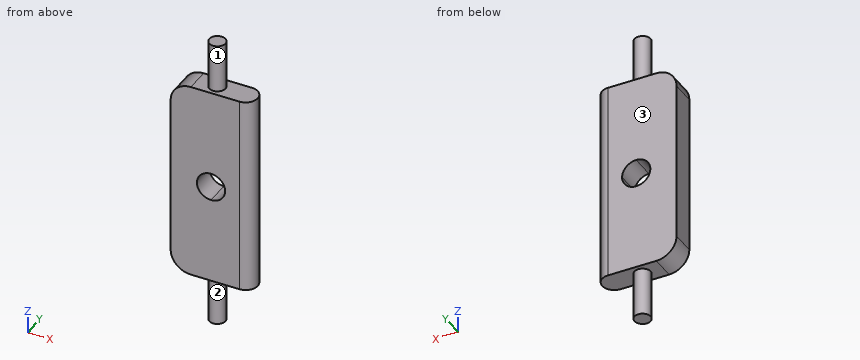
from build123d import *

# Parameters (mm, degrees)
SKETCH1_W           = 20
SKETCH1_H           = 50
BOSS_EXTRUDE1_DEPTH = 6
CUT_EXTRUDE1_DEPTH  = 55.184868737
BOSS_EXTRUDE2_DEPTH = 4
BOSS_EXTRUDE3_START = 4
BOSS_EXTRUDE3_DEPTH = 4
BOSS_EXTRUDE4_START = 1
SKETCH5_R           = 2
BOSS_EXTRUDE4_DEPTH = 1
SKETCH6_R           = 2
BOSS_EXTRUDE5_DEPTH = 1
FILLET1_R           = 5
FILLET2_R           = 5
FILLET3_RADIUS      = 3
FILLET3_LENGTH      = 50
BOSS_EXTRUDE6_START = 7
SKETCH7_R           = 2
BOSS_EXTRUDE6_DEPTH = 7
SKETCH8_R           = 2
BOSS_EXTRUDE7_DEPTH = 7


with BuildPart() as part:
    # Sketch1 → Boss-Extrude1 (new body)
    with BuildSketch(Plane(origin=(0, 0, 0), x_dir=(1, 0, 0), z_dir=(0, 1, 0))):
        with Locations((10, 25)):
            Rectangle(SKETCH1_W, SKETCH1_H)
    extrude(amount=BOSS_EXTRUDE1_DEPTH)

    # Sketch2 → Cut-Extrude1 (cut, through all)
    with BuildSketch(Plane(origin=(0, 6, 0), x_dir=(1, 0, 0), z_dir=(0, 1, 0))):
        with BuildLine():
            ThreePointArc((13.5, 25), (12.474873734, 27.474873734), (10, 28.5))
            Line((10, 28.5), (10, 21.5))
            ThreePointArc((10, 21.5), (12.474873734, 22.525126266), (13.5, 25))
        make_face()
        with BuildLine():
            Line((10, 21.5), (10, 28.5))
            ThreePointArc((10, 28.5), (6.5, 25), (10, 21.5))
        make_face()
    extrude(amount=-CUT_EXTRUDE1_DEPTH, mode=Mode.SUBTRACT)

    # Sketch3 → Boss-Extrude2 (add)
    with BuildSketch(Plane.XY):
        with BuildLine():
            ThreePointArc((12, 3), (11.414213562, 4.414213562), (10, 5))
            Line((10, 5), (10, 1))
            ThreePointArc((10, 1), (11.414213562, 1.585786438), (12, 3))
        make_face()
        with BuildLine():
            Line((10, 1), (10, 5))
            ThreePointArc((10, 5), (8, 3), (10, 1))
        make_face()
    extrude(amount=BOSS_EXTRUDE2_DEPTH)

    # Sketch4 → Boss-Extrude3 (add)
    with BuildSketch(Plane(origin=(0, 0, -50), x_dir=(-1, 0, 0), z_dir=(0, 0, -1)).offset(BOSS_EXTRUDE3_START)):
        with BuildLine():
            ThreePointArc((-8, 3), (-8.585786438, 4.414213562), (-10, 5))
            Line((-10, 5), (-10, 1))
            ThreePointArc((-10, 1), (-8.585786438, 1.585786438), (-8, 3))
        make_face()
        with BuildLine():
            Line((-10, 1), (-10, 5))
            ThreePointArc((-10, 5), (-12, 3), (-10, 1))
        make_face()
    extrude(amount=-BOSS_EXTRUDE3_DEPTH)

    # Sketch5 → Boss-Extrude4 (add)
    with BuildSketch(Plane(origin=(0, 0, -54), x_dir=(-1, 0, 0), z_dir=(0, 0, -1)).offset(BOSS_EXTRUDE4_START)):
        with Locations((-10, 3)):
            Circle(SKETCH5_R)
    extrude(amount=-BOSS_EXTRUDE4_DEPTH)

    # Sketch6 → Boss-Extrude5 (add)
    with BuildSketch(Plane.XY.offset(4)):
        with Locations(Location((10, 3, 0), (0, 0, 180))):
            Circle(SKETCH6_R)
    extrude(amount=BOSS_EXTRUDE5_DEPTH)

    # Fillet1
    fillet1_edges = [part.edges().sort_by_distance(p)[0] for p in [
        (0, 3, -50),
    ]]
    fillet(fillet1_edges, radius=FILLET1_R)

    # Fillet2
    fillet2_edges = [part.edges().sort_by_distance(p)[0] for p in [
        (0, 3, 0),
    ]]
    fillet(fillet2_edges, radius=FILLET2_R)

    # Fillet3: full round fillet: the end face becomes a half cylinder, R = half its width
    fillet3_face = Plane((20, 3, -25), x_dir=(0, 0, 1), z_dir=(1, 0, 0))  # on the end face: x along it, z out of the body
    fillet3_slab = fillet3_face.offset(-FILLET3_RADIUS / 2) * Box(FILLET3_LENGTH, 2 * FILLET3_RADIUS, FILLET3_RADIUS, mode=Mode.PRIVATE)  # the body's end, R deep
    fillet3_round = Plane((17, 3, -25), x_dir=(1, 0, 0), z_dir=(0, 0, 1)) * Cylinder(FILLET3_RADIUS, FILLET3_LENGTH, mode=Mode.PRIVATE)  # its axis R under the face
    add(fillet3_slab - fillet3_round, mode=Mode.SUBTRACT)

    # Sketch7 → Boss-Extrude6 (add)
    with BuildSketch(Plane(origin=(0, 0, -55), x_dir=(-1, 0, 0), z_dir=(0, 0, -1)).offset(BOSS_EXTRUDE6_START)):
        with Locations((-10, 3)):
            Circle(SKETCH7_R)
    extrude(amount=-BOSS_EXTRUDE6_DEPTH)

    # Sketch8 → Boss-Extrude7 (add)
    with BuildSketch(Plane.XY.offset(5)):
        with Locations(Location((10, 3, 0), (0, 0, 180))):
            Circle(SKETCH8_R)
    extrude(amount=BOSS_EXTRUDE7_DEPTH)


solid = part.part
The listing builds one solid part. Answer for the finished solid, in the listing's coordinates (mm). Face numbers are marked on the shaded views. A direction names the side the tool comes from. Give positions to 0.01 mm unless a question says otherwise; leave off trailing zeros. Write each loop counter-clockwise with the first axis right and the second up, starting at its lowest first coordinate (ties: lowest second). Pieces come first, ordered by that corner, then holes. Notation, with made-up numbers: (54, 3.25) -> (106, 3.25) arc R21 cw to (106, 28.25) -> close; hole circle Ø8 at (-7, 36.5). An arc over 180 degrees is marked (long way). One line per question, with ' | ' between items. Start each with the question number.
1. For the marked faces 1, 2 and 3, determine the directions among +Z, -Z, +X, -X, +Y, -Y from which every point of the face is accessible in a straight line to the end or side of a thin tool.
2. Section C-C (z = -56.5) is taken. Determine the outline of the cut face in (x, y), plus the area to 3 significant figures.
3. Section A-A (z = -40.5) is taken. Determine the outline of the cut face in (x, y).
4. Section B-B (x = 15) is taken. Determine the outline of the cut face in (y, z), plus the area to 3 significant figures.
5. Find the intervals of material crossed by probe 1 along X at (y, z) = (3.2, -6); probe 2 along Z at (x, y) = (5.25, 2.5); probe 3 along Z at (x, y) = (12.75, 1.7), in increasing order.
6. Given pin 1 Ø1.8 at (x, y) = (15, 4.5) entering from -Z; pin 2 Ø3 at (y, z) = (4.5, 2) entering from +X, each flat-ended and moving along its own axis, determine where each tip first touches the part or whether it passes through.
Response values:
1) face 1: +Z | face 2: -Z | face 3: +Z, -Z, +X, -X, +Y
2) outline: circle Ø4 at (10, 3) | area: 12.6 mm2
3) outline: (0, 0) -> (17, 0) arc R3 ccw to (17, 6) -> (0, 6) -> close
4) outline: (0, -50) -> (6, -50) -> (6, 0) -> (0, 0) -> close | area: 300 mm2
5) probe 1: 0 to 19.99 | probe 2: -50 to 0 | probe 3: -50 to -27.17, -22.83 to 0
6) pin 1: z = -50 | pin 2: x = 12
